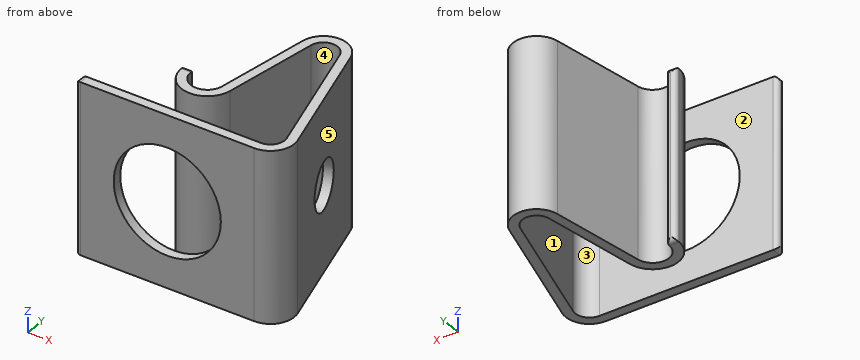
from build123d import *

# Parameters (mm, degrees)
F1_DEPTH = 72
F2_R     = 1.99999
F3_R     = 1.99999
F4_R     = 10
F5_DEPTH = 5
F8_R     = 22.5
F9_DEPTH = 5


# Not quite as in the source:
# - a fillet or chamfer is up to 0.001 mm smaller than in the source, because OpenCascade refuses the exact size
# - a feature of the source that left no trace in its solid (it failed there, or was rolled back) is left out


with BuildPart() as f1:
    # F0 (on Top) → F1 (new body)
    with BuildSketch(Plane.XY):
        with BuildLine():
            Line((-9.8480775301, 1.7364817767), (-16.7940046368, -37.6558283438))
            ThreePointArc((-16.7940046368, -37.6558283438), (-24.2977491071, -43.4136539868), (-30.6876589079, -36.4402911002))
            Line((-30.6876589079, -36.4402911002), (-30.6876589079, -34.4402911002))
            Line((-30.6876589079, -34.4402911002), (-34.6876589079, -34.4402911002))
            Line((-34.6876589079, -34.4402911002), (-34.6876589079, -36.4402911002))
            ThreePointArc((-34.6876589079, -36.4402911002), (-24.6463720781, -47.3984327792), (-12.8547736248, -38.3504210545))
            Line((-12.8547736248, -38.3504210545), (-5.9088465181, 1.041889066))
            ThreePointArc((-5.9088465181, 1.041889066), (-0.2617163242, 5.9942893295), (5.7955549577, 1.5529142706))
            Line((5.7955549577, 1.5529142706), (20.0306024384, -51.5730061753))
            ThreePointArc((20.0306024384, -51.5730061753), (18.9951675224, -56.77848902), (14.2350474806, -59.1259204459))
            Line((14.2350474806, -59.1259204459), (-60.7649525194, -59.1259204459))
            Line((-60.7649525194, -59.1259204459), (-60.7649525194, -63.1259204459))
            Line((-60.7649525194, -63.1259204459), (14.2350474806, -63.1259204459))
            ThreePointArc((14.2350474806, -63.1259204459), (22.1685808836, -59.213534736), (23.8943057435, -50.5377299949))
            Line((23.8943057435, -50.5377299949), (9.6592582629, 2.588190451))
            ThreePointArc((9.6592582629, 2.588190451), (-0.4361938737, 9.9904822158), (-9.8480775301, 1.7364817767))
        make_face()
    extrude(amount=F1_DEPTH)

    # F2 (radius 2 in the source; OpenCascade refuses exactly that, so slightly less here)
    f2_edges = [f1.edges().sort_by_distance(p)[0] for p in [
        (-30.687659, -34.440291, 36),
        (-34.687659, -34.440291, 36),
        (-32.687659, -34.440291, 0),
        (-32.687659, -34.440291, 72),
    ]]
    fillet(f2_edges, radius=F2_R)

    # F3 (radius 2 in the source; OpenCascade refuses exactly that, so slightly less here)
    f3_edges = [f1.edges().sort_by_distance(p)[0] for p in [
        (-60.764953, -59.12592, 36),
        (-60.764953, -63.12592, 36),
        (-60.764953, -61.12592, 0),
        (-60.764953, -61.12592, 72),
    ]]
    fillet(f3_edges, radius=F3_R)

    # F4 (on face) → F5 (cut)
    with BuildSketch(Plane(origin=(9.6592582629, 2.588190451, 0), x_dir=(-0.2588190451, 0.9659258263, 0), z_dir=(0.9659258263, 0.2588190451, 0))):
        with Locations((-27.5, 36)):
            Circle(F4_R)
    extrude(amount=-F5_DEPTH, mode=Mode.SUBTRACT)

    # F8 (on face) → F9 (cut)
    with BuildSketch(Plane.XZ.offset(63.1259204459)):
        with Locations((-22.2649525194, 36)):
            Circle(F8_R)
    extrude(amount=-F9_DEPTH, mode=Mode.SUBTRACT)


solid = f1.part
Build history of the part. All positions in model axes, mm. Face numbers are marked on the shaded views. A direction names the side the tool comes from. Give positions to 0.01 mm unless a question says otherwise; leave off trailing zeros. Write each loop counter-clockwise with the first axis right and the second up, starting at its lowest first coordinate (ties: lowest second). Pieces come first, ordered by that corner, then holes. Notation, with made-up numbers: (59, -39.5) - (86, -39.5) arc R16 ccw to (86, -12.5) - close; hole circle Ø1 at (81.25, -23). An arc over 180 degrees is marked (long way). Use one line per item in the form item = value. Start each with the question number.
1. 3-axis set-ups, long thin cutter, end or side, ignore diameter. For the marked faces 4 and 5: which of +Z, -Z, +X, -X, +Y, -Y reach the whole face in a straight line?
2. Two-plate mould, pull along X, no slides. Class the marked faces 1, 2 and 3: released by +X, released by -X, zero draft, split by the parting line, or undercut.
3. Band-saw the part on D-D on y = -40. Write the cut outline in (x, z).
4. Probe line 1 (Y direction, x = -36, z = 57.5); line 2 (Y direction, x = -29, z = 61); line 3 (Y direction, x = -31, z = 57). List the from-to ranges inside material, lowest first. Write a range as [from, to].
5. Band-saw the part on B-B on x = 4.5. Write the cut outline in (y, z), plus the area to 3 significant figures.
6. Band-saw the part on A-A on y = -1. Write the cut outline in (x, z).
7. Drop flat-ended pins along their axis: pin 1 Ø4 at (y, z) = (-37.5, 37) entering from -X; pin 2 Ø6 at (y, z) = (-48, 12.5) entering from +X; pin 3 Ø2 at (y, z) = (-5.5, 19) entering from -X. Give the stop position or say it passes through.
Conclusion:
q1.face_4 = +Z, -Z
q1.face_5 = +Z, -Z, +X, +Y
q2.face_1 = undercut
q2.face_2 = zero draft
q2.face_3 = released by -X
q3.outline = (-34.1, 0) - (-29.71, 0) - (-29.71, 72) - (-34.1, 72) - close; (-17.66, 0) - (-13.28, 0) - (-13.28, 72) - (-17.66, 72) - close; (16.93, 0) - (21.07, 0) - (21.07, 72) - (16.93, 72) - close
q4.line_1 = [-63.13, -59.13]
q4.line_2 = [-63.13, -59.13], [-46.07, -41]
q4.line_3 = [-63.13, -59.13], [-44.66, -35.37]
q5.outline = (-63.13, 0) - (-59.13, 0) - (-59.13, 72) - (-63.13, 72) - close; (3.97, 0) - (8.93, 0) - (8.93, 72) - (3.97, 72) - close
q5.area = 645 mm²
q6.outline = (-10.33, 0) - (-6.27, 0) - (-6.27, 72) - (-10.33, 72) - close; (6.48, 0) - (10.62, 0) - (10.62, 72) - (6.48, 72) - close
q7.pin_1 = -34.69
q7.pin_2 = 24.01
q7.pin_3 = -11.3
